The figure shows three views and two pictorial views of one solid part (mm, origin at its lowest corner). Answer the questions. A direction names the side the tool comes from. Give positions to 0.01 mm unless a question says otherwise; leave off trailing zeros. Loops run counter-clockwise (first coordinate to the right, second up) from the corner with the lowest first, then second, coordinate; pieces in that order, holes last. Notation, with made-up numbers: M 62,12.5 L 105,12.5 A27 cw 105,29.5 Z; hole C -13,34.25 d6. An arc over 180 degrees is marked long. Answer as a JSON object with one key per item and string values. Group by question number.
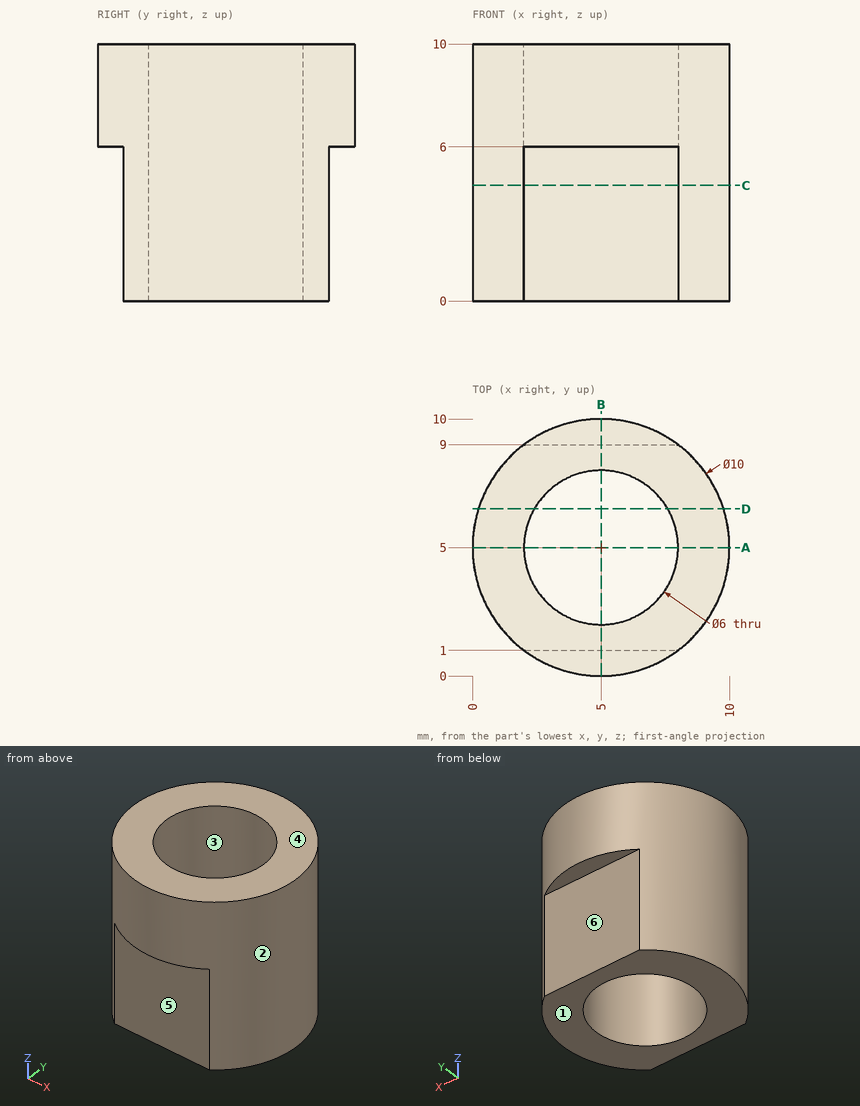
Item 1: A cutting plane is placed at A-A (y = 5). Determine the outline of the cut face in (x, z), and give its area (3 significant figures).
Item 2: Given pin 1 Ø4 at (x, y) = (7, 7) entering from +Z; pin 2 Ø1.5 at (y, z) = (2, 2.5) entering from +X; pin 3 Ø0.8 at (x, y) = (4, 9.5) entering from -Z; pin 4 Ø3 at (x, z) = (4, 3) entering from -Y, each flat-ended and moving along its own axis, determine where each tip first touches the part or whether it passes through.
Item 3: Find the intervals of material crossed by probe 1 along Y at (x, z) = (5, 6.25); probe 2 along Y at (x, z) = (5, 3.25); probe 3 along X at (y, z) = (2.5, 3), in increasing order. Write a range as [from, to].
Item 4: A cutting plane is placed at B-B (x = 5). Determine the outline of the cut face in (y, z), and give its area (3 significant figures).
Item 5: A cutting plane is placed at D-D (y = 6.5). Determine the outline of the cut face in (x, z), and give its area (3 significant figures).
Item 6: A cutting plane is placed at C-C (z = 4.5). Determine the outline of the cut face in (x, y), and give its area (3 significant figures).
Item 7: A tool of negligible diameter and unlimited length cuts with its end or side. For the marked faces 4, 5 and 6, from which of +Z, -Z, +X, -X, +Y, -Y can it reach the whole face along a straight path? Write none if from no direction.
Item 8: For a pull along Y with two mould halves and no side action, classify the marked faces 1, 2 and 3 as pulls with the +Y half, pulls with the -Y half, needs draft (parallel to the pull), parting line crosses it, or undercut.
The answers:
{
 "1": {"outline": "M 0,0 L 2,0 L 2,10 L 0,10 Z; M 8,0 L 10,0 L 10,10 L 8,10 Z", "area": "40.0 mm^2"},
 "2": {"pin 1": "stops at z = 10", "pin 2": "stops at x = 9.47", "pin 3": "stops at z = 6", "pin 4": "stops at y = 1"},
 "3": {"probe 1": "y = [0, 2], [8, 10]", "probe 2": "y = [1, 2], [8, 9]", "probe 3": "x = [0.67, 3.34], [6.66, 9.33]"},
 "4": {"outline": "M 0,6 L 1,6 L 1,0 L 2,0 L 2,10 L 0,10 Z; M 8,0 L 9,0 L 9,6 L 10,6 L 10,10 L 8,10 Z", "area": "28.0 mm^2"},
 "5": {"outline": "M 0.23,0 L 2.4,0 L 2.4,10 L 0.23,10 Z; M 7.6,0 L 9.77,0 L 9.77,10 L 7.6,10 Z", "area": "43.4 mm^2"},
 "6": {"outline": "M 2,1 L 8,1 A5 ccw 8,9 L 2,9 A5 ccw Z; hole C 5,5 d6", "area": "42.1 mm^2"},
 "7": {"face 4": "+Z, +X, -X, +Y, -Y", "face 5": "-Z, +X, -X, -Y", "face 6": "-Z, +X, -X, +Y"},
 "8": {"face 1": "needs draft", "face 2": "parting line crosses it", "face 3": "undercut"}
}
